from build123d import *

# Parameters (mm, degrees)
CYLINDER_R           = 15
CYLINDER_DEPTH       = 100
CYLINDER_PITCH_ANGLE = 90
BOX005_W             = 100
BOX005_H             = 30
BOX005_DEPTH         = 30
BOX004_W             = 40
BOX004_H             = 40
BOX004_DEPTH         = 120
BOX004_ROLL_ANGLE    = -5.2
BOX003_W             = 40
BOX003_H             = 40
BOX003_DEPTH         = 120
BOX003_ROLL_ANGLE    = 5.2
BOX001_W             = 19
BOX001_H             = 100
BOX001_DEPTH         = 110
BOX001_PITCH_ANGLE   = 8.4
BOX_W                = 25
BOX_H                = 80
BOX_DEPTH            = 100


with BuildPart() as cylinder:
    # Cylinder → Cylinder (new body)
    with BuildSketch(Plane.XY):
        Circle(CYLINDER_R)
    extrude(amount=CYLINDER_DEPTH)


with BuildPart() as cylinder_1:
    # Cylinder pitch: moved
    add(cylinder.part.rotate(Axis((0, 0, 0), (0, 1, 0)), CYLINDER_PITCH_ANGLE))


with BuildPart() as cylinder_2:
    # Cylinder placement: moved
    add(cylinder_1.part.moved(Location((0, 40, 70))))


with BuildPart() as fusion:
    # Box005 → Box005 (new body)
    with BuildSketch(Plane(origin=(0, 25, 70), x_dir=(1, 0, 0), z_dir=(0, 0, 1))):
        with Locations((50, 15)):
            Rectangle(BOX005_W, BOX005_H)
    extrude(amount=BOX005_DEPTH)

    # Fusion: union Cylinder
    add(cylinder_2.part)


with BuildPart() as cube002:
    # Box004 → Box004 (new body)
    with BuildSketch(Plane.XY):
        with Locations((20, 20)):
            Rectangle(BOX004_W, BOX004_H)
    extrude(amount=BOX004_DEPTH)


with BuildPart() as cube002_1:
    # Box004 roll: moved
    add(cube002.part.rotate(Axis((0, 0, 0), (1, 0, 0)), BOX004_ROLL_ANGLE))


with BuildPart() as cube002_2:
    # Box004 placement: moved
    add(cube002_1.part.moved(Location((0, 70, -4))))


with BuildPart() as cube003:
    # Box003 → Box003 (new body)
    with BuildSketch(Plane.XY):
        with Locations((20, 20)):
            Rectangle(BOX003_W, BOX003_H)
    extrude(amount=BOX003_DEPTH)


with BuildPart() as cube003_1:
    # Box003 roll: moved
    add(cube003.part.rotate(Axis((0, 0, 0), (1, 0, 0)), BOX003_ROLL_ANGLE))


with BuildPart() as cube003_2:
    # Box003 placement: moved
    add(cube003_1.part.moved(Location((0, -30, -4))))


with BuildPart() as cube001:
    # Box001 → Box001 (new body)
    with BuildSketch(Plane.XY):
        with Locations((9.5, 50)):
            Rectangle(BOX001_W, BOX001_H)
    extrude(amount=BOX001_DEPTH)


with BuildPart() as cube001_1:
    # Box001 pitch: moved
    add(cube001.part.rotate(Axis((0, 0, 0), (0, 1, 0)), BOX001_PITCH_ANGLE))


with BuildPart() as cube001_2:
    # Box001 placement: moved
    add(cube001_1.part.moved(Location((10, 0, 0))))


with BuildPart() as cut003:
    # Box → Box (new body)
    with BuildSketch(Plane.XY):
        with Locations((12.5, 40)):
            Rectangle(BOX_W, BOX_H)
    extrude(amount=BOX_DEPTH)

    # Cut: cut Cube001
    add(cube001_2.part, mode=Mode.SUBTRACT)

    # Cut001: cut Cube003
    add(cube003_2.part, mode=Mode.SUBTRACT)

    # Cut002: cut Cube002
    add(cube002_2.part, mode=Mode.SUBTRACT)

    # Cut003: cut Fusion
    add(fusion.part, mode=Mode.SUBTRACT)


solid = cut003.part
Could you check a few things on this model? Use its own coordinates, in mm. A direction names the side the tool comes from. Coordinates: 2 decimals unless noted, no trailing zeros. Order: outer loops, then holes, each group sorted by start corner. A loop starts at its lowest first (then second) coordinate and runs counter-clockwise, first axis right, second up.
Q1. Which directions (+Z, -Z, +X, -X, +Y, -Y) give clear straight access to the entire face, cutting with the end or side of a thin tool? Please do faces 1 (the flat face through (0, 40, 49)), 2 (the flat face through (12, 25, 85)).
Q2. Suppose I cut it at C-C on z = 12. Please give me the cut outline in (x, y), and give its area (3 significant figures).
Q3. Suppose I cut it at B-B on y = 13. Please give me the cut outline in (x, z).
Q4. Thinking about a two-plate mould opening in Y: for faces 3 (the flat face through (12, 55, 85)), 4 (the flat face through (17.28, 39.53, 49.3)), 5 (the flat face through (9.46, 75.86, 60.41)), which applies, released by +Y, released by -Y, zero draft, split by the parting line, or undercut?
Q5. Suppose I cut it at D-D on x = 12. Please give me the cut outline in (y, z).
Q6. Suppose I cut it at A-A on x = 3. Please give me the cut outline in (y, z), and give its area (3 significant figures).
Q7. Will these pins go through, and if not, where does the flat tip stop? pin 1 (1.5 mm diameter, centred on x = 7.5, z = 29, fed in from -Y); pin 2 (3 mm diameter, centred on x = 4, z = 53, fed in from -Y); pin 3 (7.5 mm diameter, centred on x = 11, z = 84, fed in from +Y).
Q8. Please list where these lines run through material, in increasing order: L1, parallel to Y at x = 12.75, z = 62; L2, parallel to Y at x = 11, z = 60.5; L3, parallel to Y at x = 8.75, z = 44.
Answer:
1. face 1: +Z, -Z, -X, +Y, -Y
1. face 2: +Z, +X, -X
2. outline: (0, 8.71) - (11.77, 8.71) - (11.77, 71.46) - (0, 71.46) - close
2. area: 739 mm2
3. outline: (0, 0) - (10, 0) - (24.77, 100) - (0, 100) - close
4. face 3: undercut
4. face 4: zero draft
4. face 5: released by +Y
5. outline: (0.7, 100) - (8.57, 13.54) - (71.6, 13.54) - (79.46, 100) - (55, 100) - (55, 70) arc R15 cw to (25, 70) - (25, 100) - close
6. outline: (0.7, 100) - (9.8, 0) - (70.36, 0) - (79.46, 100) - (55, 100) - (55, 70) arc R15 cw to (25, 70) - (25, 100) - close
6. area: 5,710 mm2
7. pin 1: stops at y = 7.09
7. pin 2: stops at y = 4.84
7. pin 3: stops at y = 78.35
8. L1: y = 4.16 to 27.31, 52.69 to 76.01
8. L2: y = 4.3 to 28.39, 51.61 to 75.87
8. L3: y = 5.8 to 74.37
